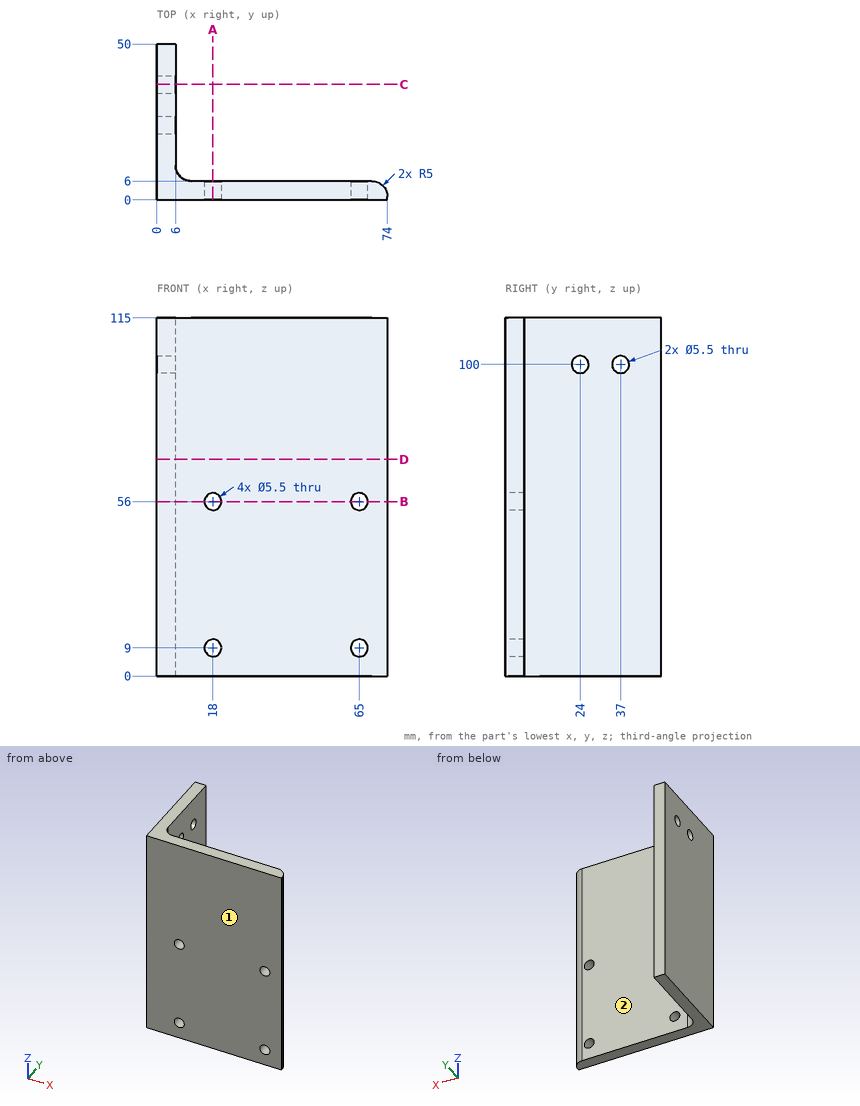
Drawing for the job (mm, zero at the part's lowest x, y, z). A direction names the side the tool comes from. Round coordinates to 2 decimals unless told otherwise and drop trailing zeros. Write each loop counter-clockwise with the first axis right and the second up, starting at its lowest first coordinate (ties: lowest second). Pieces come first, ordered by that corner, then holes. Notation, with made-up numbers: M -37.5,59 L -10.5,59 A33 cw -10.5,87 Z; hole C 58.25,60.25 d9. An arc over 180 degrees is marked long. Answer as a JSON object with one key per item and string values. Group by question number.
(1) Drill centre lines: L1, parallel to Z at x = 65, y = 3.15; L2, parallel to Y at x = 3, z = 100; L3, parallel to X at y = 33, z = 95. Where is each one in solid material? Low to high.
(2) Flat gauge pins, fed straight in: pin 1 (17.5 mm diameter, centred on x = 48, z = 42.5, fed in from +Y); pin 2 (7 mm diameter, centred on y = 24, z = 100, fed in from +X); pin 3 (6 mm diameter, centred on y = 8, z = 47.5, fed in from +X). Where does each tip first touch, or does it go through?
(3) Which spindle directions (+Z, -Z, +X, -X, +Y, -Y) get a long thin tool onto all of the face, cutting with end or side? Do the marked faces 1 and 2. Say none if no direction does.
(4) Cut at B-B (z = 56). Give the cut face in (x, y).
(5) Cut at A-A (x = 18). Give the cut face in (y, z), and give its area (3 significant figures).
(6) Cut at C-C (y = 37). Give the cut face in (x, z).
(7) Cut at D-D (z = 69.5). Give the cut face in (x, y).
Responses:
{
 "1": {"L1": "z = 0 to 6.25, 11.75 to 53.25, 58.75 to 115", "L2": "y = 0 to 21.25, 26.75 to 34.25, 39.75 to 50", "L3": "x = 0 to 6"},
 "2": {"pin 1": "stops at y = 6", "pin 2": "stops at x = 6", "pin 3": "stops at x = 72"},
 "3": {"face 1": "+Z, -Z, +X, -X, -Y", "face 2": "+Z, -Z, +X, +Y"},
 "4": {"outline": "M 0,0 L 15.25,0 L 15.25,6 L 11,6 A5 cw 6,11 L 6,50 L 0,50 Z; M 20.75,0 L 62.25,0 L 62.25,6 L 20.75,6 Z; M 67.75,0 L 74,0 L 74,1 A5 ccw 69,6 L 67.75,6 Z"},
 "5": {"outline": "M 0,0 L 6,0 L 6,6.25 L 0,6.25 Z; M 0,11.75 L 6,11.75 L 6,53.25 L 0,53.25 Z; M 0,58.75 L 6,58.75 L 6,115 L 0,115 Z", "area": "624 mm2"},
 "6": {"outline": "M 0,0 L 6,0 L 6,97.25 L 0,97.25 Z; M 0,102.75 L 6,102.75 L 6,115 L 0,115 Z"},
 "7": {"outline": "M 0,0 L 74,0 L 74,1 A5 ccw 69,6 L 11,6 A5 cw 6,11 L 6,50 L 0,50 Z"}
}
